Geometry check sheet. Reference: the model listing, model coordinates, mm. Face numbers are marked on the shaded views. Round coordinates to 2 decimals unless told otherwise and drop trailing zeros. Write each loop counter-clockwise with the first axis right and the second up, starting at its lowest first coordinate (ties: lowest second). Pieces come first, ordered by that corner, then holes. Notation, with made-up numbers: (-34, 1.25) - (5, 1.25) arc R26 cw to (5, 23.25) - close; hole circle Ø3 at (65, 82). An arc over 180 degrees is marked (long way). Return JSON: item names as keys, results as strings.
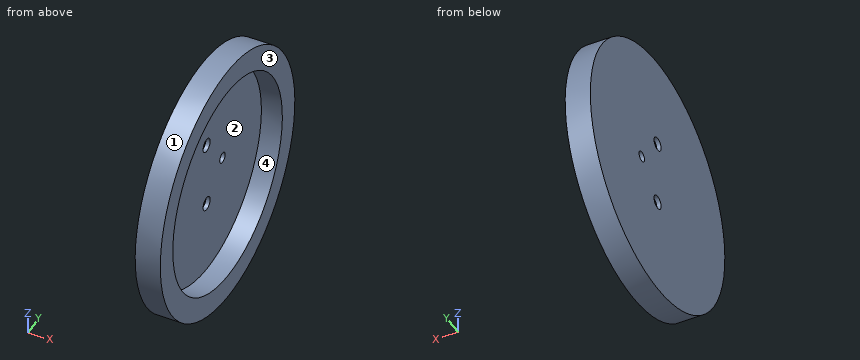
```python
from build123d import *

# Parameters (mm, degrees)
SKETCH2_R           = 62
BOSS_EXTRUDE1_DEPTH = 12
SKETCH4_R           = 50.5
CUT_EXTRUDE2_DEPTH  = 10
SKETCH5_R           = 2.5
SKETCH5_R_2         = 3.25
CUT_EXTRUDE3_DEPTH  = 5


with BuildPart() as part:
    # Sketch2 → Boss-Extrude1 (new body)
    with BuildSketch(Plane(origin=(0, 0, 0), x_dir=(0, 0, -1), z_dir=(1, 0, 0))):
        Circle(SKETCH2_R)
    extrude(amount=BOSS_EXTRUDE1_DEPTH)

    # Sketch4 → Cut-Extrude2 (cut)
    with BuildSketch(Plane(origin=(12, 0, 0), x_dir=(0, 0, -1), z_dir=(1, 0, 0))):
        Circle(SKETCH4_R)
    extrude(amount=-CUT_EXTRUDE2_DEPTH, mode=Mode.SUBTRACT)

    # Sketch5 → Cut-Extrude3 (cut)
    with BuildSketch(Plane.ZY):
        with Locations((0, 14.581539196)):
            Circle(SKETCH5_R)
        with Locations((-14.480976857, 0)):
            Circle(SKETCH5_R_2)
        with Locations((17.497847035, 0)):
            Circle(SKETCH5_R_2)
    extrude(amount=-CUT_EXTRUDE3_DEPTH, mode=Mode.SUBTRACT)


solid = part.part
```
(1) Gauge pin test, flat ends, axial feed: pin 1 (10.5 mm diameter, centred on y = 0, z = -14.48, fed in from +X); pin 2 (5 mm diameter, centred on x = 10.5, z = -4, fed in from +Y); pin 3 (1 mm diameter, centred on x = 7, y = -43.5, fed in from -Z); pin 4 (5 mm diameter, centred on y = 0, z = 17.5, fed in from -X). Record the tip position at first contact, or that the pin passes through.
Response values:
{"pin 1": "stops at x = 2", "pin 2": "stops at y = 61.98", "pin 3": "stops at z = -44.67", "pin 4": "passes through"}
(2) Release check for a two-part mould opening along Z. For the marked faces 1, 2, 3 and 4 record: pulls with the +Z half, pulls with the -Z half, needs draft (parallel to the pull), parting line crosses it, or undercut.
Response values:
{"face 1": "parting line crosses it", "face 2": "undercut", "face 3": "needs draft", "face 4": "undercut"}
(3) Section check B-B, the plane y = 0. Enter the section's corners in (x, z).
Response values:
{"outline": "(0, -62) - (12, -62) - (12, -50.5) - (2, -50.5) - (2, -17.73) - (0, -17.73) - close; (0, -11.23) - (2, -11.23) - (2, 14.25) - (0, 14.25) - close; (0, 20.75) - (2, 20.75) - (2, 50.5) - (12, 50.5) - (12, 62) - (0, 62) - close"}
(4) Section check D-D, the plane y = 47.5. Enter the section's corners in (x, z).
Response values:
{"outline": "(0, -39.85) - (12, -39.85) - (12, -17.15) - (2, -17.15) - (2, 17.15) - (12, 17.15) - (12, 39.85) - (0, 39.85) - close"}
(5) Material ranges on line 1 along X through (y, z) = (-46.5, -15.5); line 2 along Z through (x, y) = (3, -3); line 3 along Y through (x, z) = (4.25, 38), recorded low to high. Write a range as [from, to].
Response values:
{"line 1": "x = [0, 2]", "line 2": "z = [-61.93, -50.41], [50.41, 61.93]", "line 3": "y = [-48.99, -33.26], [33.26, 48.99]"}
(6) Section check A-A, the plane z = 0. Enter the section's corners in (x, y).
Response values:
{"outline": "(0, -62) - (12, -62) - (12, -50.5) - (2, -50.5) - (2, 12.08) - (0, 12.08) - close; (0, 17.08) - (2, 17.08) - (2, 50.5) - (12, 50.5) - (12, 62) - (0, 62) - close"}
(7) Section check C-C, the plane x = 3.5. Enter the section's corners in (y, z), plus the area to 3 significant figures.
Response values:
{"outline": "circle Ø124 at (0, 0); hole circle Ø101 at (0, 0)", "area": "4,060 mm^2"}
